Read the model definition and answer for the solid it produces. Units are mm, in the model's axes. Face numbers are marked on the shaded views. A direction names the side the tool comes from. Coordinates: 2 decimals unless noted, no trailing zeros. Loops run counter-clockwise (first coordinate to the right, second up) from the corner with the lowest first, then second, coordinate; pieces in that order, holes last. Notation, with made-up numbers: (-5.75, 17) -> (10.25, 17) arc R24 ccw to (10.25, 41) -> close; hole circle Ø6 at (-20.75, 81). An arc over 180 degrees is marked (long way). Answer as a JSON object with one key per item and string values. Group by question number.
Q1. For the marked faces 1 and 2, determine the directions among +Z, -Z, +X, -X, +Y, -Y from which every point of the face is accessible in a straight line to the end or side of a thin tool.
Q2. The part is cut by section A-A on x = 77. Write down the section's boundary in (y, z), and give its area (3 significant figures).
Q3. Straight lines are drawn through the part: line 1 along Y through (x, z) = (69, 15); line 2 along X through (y, z) = (-14.5, 9.5); line 3 along X through (y, z) = (-27.5, 18). For each, find the intervals that lie inside material, in ascending order. Write a range as [from, to].
Q4. The part is cut by section B-B on y = -15. Write down the section's boundary in (x, z), and give its area (3 significant figures).
Q5. The part is cut by section C-C on z = 21.5. Write down the section's boundary in (x, y).
Q6. Each of these flat-tipped pins is pushed along its axis until it touches: P1, Ø1.5, axis at y = -34, z = 16, coming from the +X side; P2, Ø1, axis at y = -8.5, z = 11, coming from the +X side; P3, Ø3, axis at y = -29.5, z = 10.5, coming from the +X side. Where does it stop, or does it pass through?
Q7. The part is cut by section D-D on x = 55. Write down the section's boundary in (y, z).
Q8. Determine the mould class of the marked faces 3, 4, 5 and 6 for opening direction Y: released by +Y, released by -Y, zero draft, split by the parting line, or undercut.
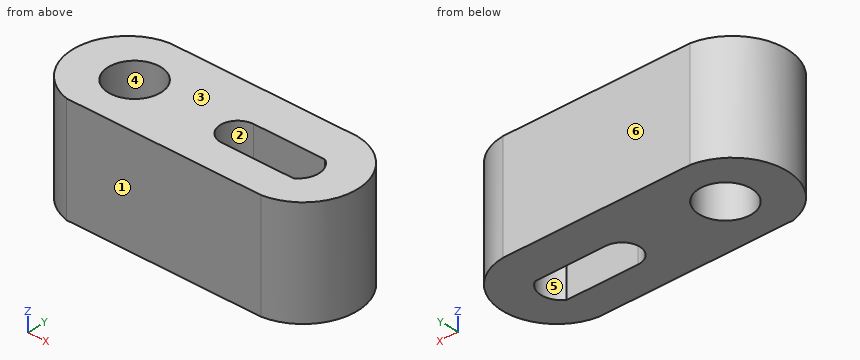
from build123d import *

# Parameters (mm, degrees)
F0_W     = 101.6
F0_H     = 38.1
F1_DEPTH = 38.1
F3_DEPTH = 38.1
F4_R     = 9.279541
F5_DEPTH = 38.1
F7_DEPTH = 101.6


with BuildPart() as f1:
    # F0 (on Front) → F1 (new body)
    with BuildSketch(Plane.XZ):
        with Locations((50.8, 19.05)):
            Rectangle(F0_W, F0_H)
    extrude(amount=F1_DEPTH)

    # F2 (on face) → F3 (cut)
    with BuildSketch(Plane.XY.offset(38.1)):
        with BuildLine():
            ThreePointArc((83.914571, 0), (101.325868, -18.794907), (84.482022, -38.1))
            Line((84.482022, -38.1), (101.6, -38.1))
            Line((101.6, -38.1), (101.6, 0))
            Line((101.6, 0), (83.914571, 0))
        make_face()
        with BuildLine():
            Line((0, -38.1), (15.216109, -38.1))
            ThreePointArc((15.216109, -38.1), (0.393633, -18.225575), (17.202171, 0))
            Line((17.202171, 0), (0, 0))
            Line((0, 0), (0, -38.1))
        make_face()
    extrude(amount=-F3_DEPTH, mode=Mode.SUBTRACT)

    # F4 (on face) → F5 (cut)
    with BuildSketch(Plane.XY.offset(38.1)):
        with Locations((22.343248, -19.372153)):
            Circle(F4_R)
    extrude(amount=-F5_DEPTH, mode=Mode.SUBTRACT)

    # F6 (on face) → F7 (cut)
    with BuildSketch(Plane.XY.offset(38.1)):
        with BuildLine():
            Line((85.293495, -14.016386), (59.893495, -14.016386))
            ThreePointArc((59.893495, -14.016386), (53.719888, -20.189993), (59.893495, -26.363599))
            Line((59.893495, -26.363599), (85.293495, -26.363599))
            ThreePointArc((85.293495, -26.363599), (88.674518, -20.189993), (85.293495, -14.016386))
        make_face()
    extrude(amount=-F7_DEPTH, mode=Mode.SUBTRACT)


solid = f1.part
Final values:
{
 "1": {"face 1": "+Z, -Z, +X, -X, -Y", "face 2": "+Z, -Z"},
 "2": {"outline": "(-38.1, 0) -> (-26.36, 0) -> (-26.36, 38.1) -> (-38.1, 38.1) -> close; (-14.02, 0) -> (0, 0) -> (0, 38.1) -> (-14.02, 38.1) -> close", "area": "981 mm2"},
 "3": {"line 1": "y = [-38.1, -26.36], [-14.02, 0]", "line 2": "x = [0.95, 14.45], [30.24, 57.5], [85.96, 100.77]", "line 3": "x = [2.21, 17.87], [26.82, 99.38]"},
 "4": {"outline": "(0.84, 0) -> (14.16, 0) -> (14.16, 38.1) -> (0.84, 38.1) -> close; (30.53, 0) -> (56.55, 0) -> (56.55, 38.1) -> (30.53, 38.1) -> close; (86.52, 0) -> (100.89, 0) -> (100.89, 38.1) -> (86.52, 38.1) -> close", "area": "2,050 mm2"},
 "5": {"outline": "(15.22, -38.1) -> (84.48, -38.1) arc R19.16 ccw to (83.91, 0) -> (17.2, 0) arc R19.41 ccw to start; hole circle Ø18.56 at (22.34, -19.37); hole (59.89, -26.36) -> (85.29, -26.36) arc R7.33 ccw to (85.29, -14.02) -> (59.89, -14.02) arc R6.17 ccw to start"},
 "6": {"P1": "stops at x = 95.06", "P2": "stops at x = 98.46", "P3": "stops at x = 99.13"},
 "7": {"outline": "(-38.1, 0) -> (-23.95, 0) -> (-23.95, 38.1) -> (-38.1, 38.1) -> close; (-16.43, 0) -> (0, 0) -> (0, 38.1) -> (-16.43, 38.1) -> close"},
 "8": {"face 3": "zero draft", "face 4": "undercut", "face 5": "undercut", "face 6": "released by +Y"}
}
